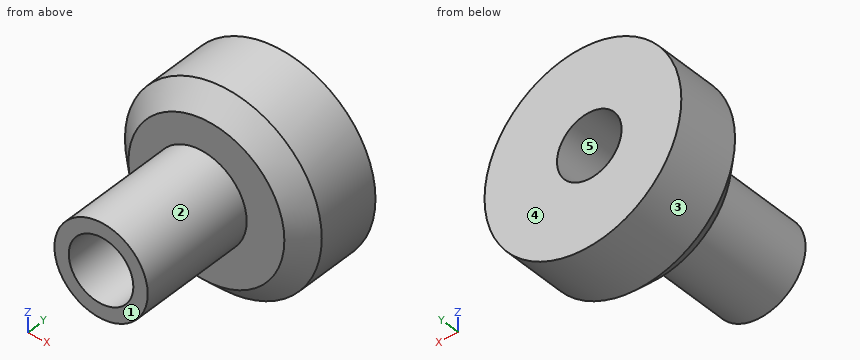
from build123d import *

# Parameters (mm, degrees)
F0_R     = 73.396839
F1_DEPTH = 63.5
F2_SIZE  = 15.24
F3_R     = 34.79629
F4_DEPTH = 88.9
F5_R     = 24.08748
F6_DEPTH = 263.398


with BuildPart() as f1:
    # F0 (on Front) → F1 (new body)
    with BuildSketch(Plane.XZ):
        Circle(F0_R)
    extrude(amount=F1_DEPTH)

    # F2
    f2_edges = [f1.edges().sort_by_distance(p)[0] for p in [
        (-73.396839, -63.5, 0),
    ]]
    chamfer(f2_edges, length=F2_SIZE)

    # F3 (on face) → F4 (join)
    with BuildSketch(Plane.XZ.offset(63.5)):
        with Locations((-4.750563, 0)):
            Circle(F3_R)
    extrude(amount=F4_DEPTH)

    # F5 (on face) → F6 (cut)
    with BuildSketch(Plane.XZ.offset(152.4)):
        with Locations((-4.750563, 0)):
            Circle(F5_R)
    extrude(amount=-F6_DEPTH, mode=Mode.SUBTRACT)


solid = f1.part
Could you check a few things on this model? Use its own coordinates, in mm. Face numbers are marked on the shaded views. A direction names the side the tool comes from. Coordinates: 2 decimals unless noted, no trailing zeros. Loops run counter-clockwise (first coordinate to the right, second up) from the corner with the lowest first, then second, coordinate; pieces in that order, holes last.
1. For the marked faces 1 and 2, which set-ups out of +Z, -Z, +X, -X, +Y, -Y let a thin tool reach every point of the face, with its end or its side?
2. Imagine slicing it at D-D (y = -58). Please give me the cut outline in (x, z), and give its area (3 significant figures).
3. I need wall thicknesses on L1, parallel to X at y = -82, z = -1; L2, parallel to Y at x = 25, z = -27; L3, parallel to Z at x = -26.5, y = -8. Which ranges of each line are inside material? Lowest first, please.
4. Imagine slicing it at A-A (z = 0). Please give me the cut outline in (x, y).
5. Imagine slicing it at B-B (y = -141). Please give me the cut outline in (x, z).
6. We'd pull the mould along Z, two halves only. Please class the marked faces 3, 4 and 5: released by +Z, released by -Z, zero draft, split by the parting line, or undercut.
7. For P1, Ø4, axis at y = -34, z = -23.5, coming from the -X side; P2, Ø3, axis at x = 57.5, y = -27.5, coming from the -Z side; P3, Ø10, axis at x = 35, z = -14, coming from the -Y side, each with a flat end and sliding along its axis, tell me the tip position at first contact or that it passes through.
8. Imagine slicing it at C-C (x = 0). Please give me the cut outline in (y, z).
Computed values:
1. face 1: +Z, -Z, +X, -X, -Y
1. face 2: -Y
2. outline: circle Ø127.31 at (0, 0); hole circle Ø48.17 at (-4.75, 0)
2. area: 10,900 mm2
3. L1: x = -39.53 to -28.82, 19.32 to 30.03
3. L2: y = -63.5 to 0
3. L3: z = -68.45 to -10.35, 10.35 to 68.45
4. outline: (-73.4, -48.26) - (-58.16, -63.5) - (-39.55, -63.5) - (-39.55, -152.4) - (-28.84, -152.4) - (-28.84, 0) - (-73.4, 0) - close; (19.34, -152.4) - (30.05, -152.4) - (30.05, -63.5) - (58.16, -63.5) - (73.4, -48.26) - (73.4, 0) - (19.34, 0) - close
5. outline: circle Ø69.59 at (-4.75, 0); hole circle Ø48.17 at (-4.75, 0)
6. face 3: split by the parting line
6. face 4: zero draft
6. face 5: undercut
7. P1: stops at x = -70.18
7. P2: stops at z = -47.45
7. P3: stops at y = -63.5
8. outline: (-152.4, -34.47) - (-63.5, -34.47) - (-63.5, -58.16) - (-48.26, -73.4) - (0, -73.4) - (0, -23.61) - (-152.4, -23.61) - close; (-152.4, 23.61) - (0, 23.61) - (0, 73.4) - (-48.26, 73.4) - (-63.5, 58.16) - (-63.5, 34.47) - (-152.4, 34.47) - close
